Drawing for the job (mm, zero at the part's lowest x, y, z). A direction names the side the tool comes from. Give positions to 0.01 mm unless a question says otherwise; leave off trailing zeros. Loops run counter-clockwise (first coordinate to the right, second up) from the corner with the lowest first, then second, coordinate; pieces in that order, holes last.
1) Wall check: line 1 (X direction, y = 45, z = 96); line 2 (X direction, y = 36, z = 150.5); line 3 (Z direction, x = 113, y = 17.5). Give the ranges that are in metal, low to high.
2) Band-saw the part on B-B on z = 11. List the corners of the cut face in (x, y), then the cut area to 3 significant figures.
3) Two-plate mould, pull along Y, no slides. Class the marked faces 5, 6 and 7: +Y half, -Y half, draft (parallel to the pull), parting line (faces both ways), or undercut.
4) Flat gauge pins, fed straight in: P1, Ø9, axis at y = 31, z = 147, coming from the +X side; P2, Ø6, axis at y = 30, z = 115.5, coming from the -X side; P3, Ø17.5, axis at x = 42.5, z = 140, coming from the +Y side. Where does each tip first touch, or does it go through?
5) Band-saw the part on A-A on x = 77. List the corners of the cut face in (y, z).
6) 3-axis set-ups, long thin cutter, end or side, ignore diameter. For the marked faces 1, 2, 3 and 4: which of +Z, -Z, +X, -X, +Y, -Y reach the whole face in a straight line?
7) Band-saw the part on D-D on x = 60. List the corners of the cut face in (y, z).
8) Band-saw the part on C-C on y = 36. State how many separate pieces and enclosed holes the cut face has, then the cut area to 3 significant figures.
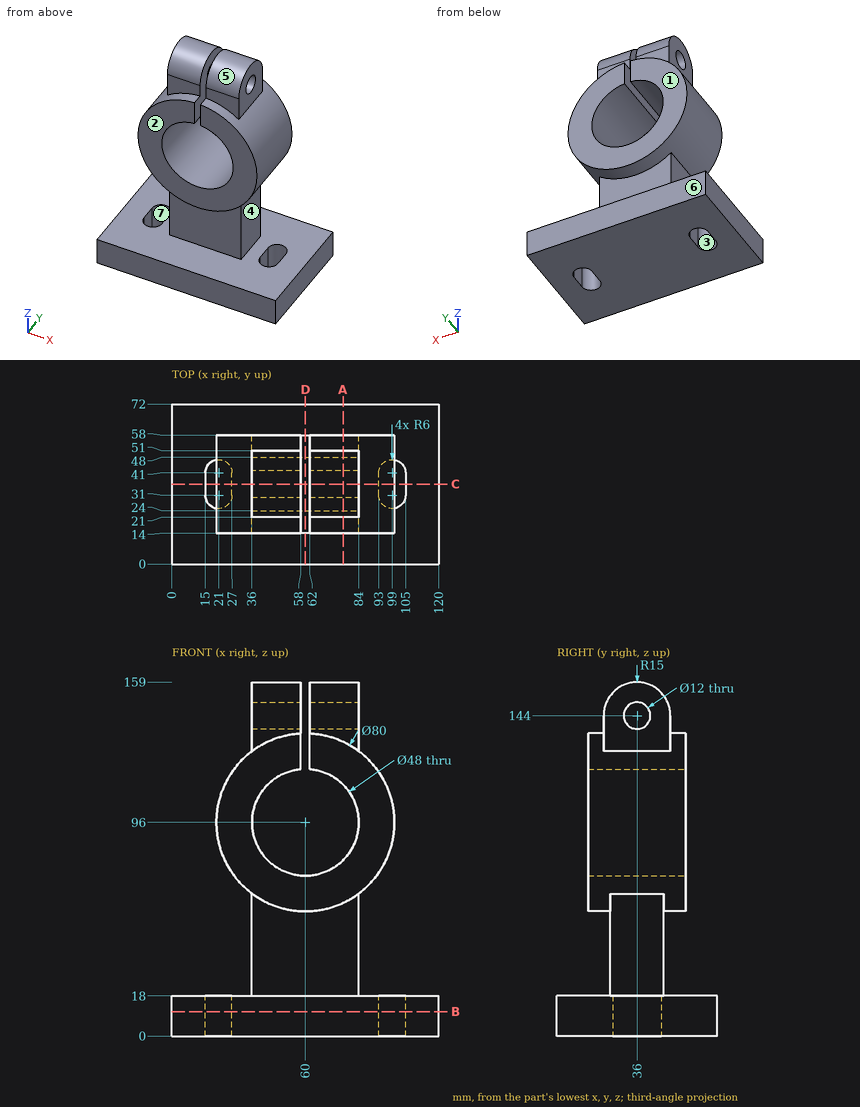
Findings below:
1. line 1: x = 20 to 36, 84 to 100
1. line 2: x = 36 to 58, 62 to 84
1. line 3: z = 0 to 18
2. outline: (0, 0) - (120, 0) - (120, 72) - (0, 72) - close; hole (15, 31) arc R6 ccw to (27, 31) - (27, 41) arc R6 ccw to (15, 41) - close; hole (93, 31) arc R6 ccw to (105, 31) - (105, 41) arc R6 ccw to (93, 41) - close
2. area: 8,170 mm2
3. face 5: parting line
3. face 6: +Y half
3. face 7: undercut
4. P1: stops at x = 84
4. P2: stops at x = 23.56
4. P3: stops at y = 58
5. outline: (0, 0) - (72, 0) - (72, 18) - (48, 18) - (48, 59.79) - (58, 59.79) - (58, 79.06) - (14, 79.06) - (14, 59.79) - (24, 59.79) - (24, 18) - (0, 18) - close; (14, 112.94) - (58, 112.94) - (58, 132.21) - (51, 132.21) - (51, 144) arc R15 ccw to (21, 144) - (21, 132.21) - (14, 132.21) - close; hole circle Ø12 at (36, 144)
6. face 1: +Z, +X, -X, +Y
6. face 2: +Z, +X, -X, -Y
6. face 3: -Z
6. face 4: +X, +Y, -Y
7. outline: (0, 0) - (72, 0) - (72, 18) - (48, 18) - (48, 56) - (58, 56) - (58, 72) - (14, 72) - (14, 56) - (24, 56) - (24, 18) - (0, 18) - close
8. separate pieces: 5
8. enclosed holes: 0
8. area: 7,430 mm2
